```python
from build123d import *

# Parameters (mm, degrees)
REVOLUTION_ANGLE = -357
SKETCH002_R      = 19.5
POCKET_DEPTH     = 36.501
POCKET001_DEPTH  = 15
CHAMFER_SIZE     = 0.25
CHAMFER001_SIZE  = 0.5
CHAMFER002_SIZE  = 0.5
CHAMFER003_SIZE  = 1


with BuildPart() as part:
    # Sketch → Revolution (revolve)
    with BuildSketch(Plane(origin=(0, 0, 0), x_dir=(0, 0, -1), z_dir=(0, -1, 0))):
        Polygon((-36.5, 0), (0, 0), (0, -21.5), (-19.5, -21.5), (-19.5, -26), (-36.5, -26), align=None)
    revolve(axis=Axis((0, 0, 0), (0, 0, -1)), revolution_arc=REVOLUTION_ANGLE)

    # Sketch002 → Pocket (cut, through all)
    with BuildSketch(Plane.XY):
        Circle(SKETCH002_R)
    extrude(amount=POCKET_DEPTH, mode=Mode.SUBTRACT)

    # Sketch001 → Pocket001 (cut)
    with BuildSketch(Plane.XY.offset(36.5)):
        with BuildLine():
            ThreePointArc((-15.975, 16.475), (-16.828553, 16.828553), (-16.475, 15.975))
            Line((-16.475, -15.975), (-16.475, 15.975))
            ThreePointArc((-16.475, -15.975), (-16.828553, -16.828553), (-15.975, -16.475))
            Line((15.975, -16.475), (-15.975, -16.475))
            ThreePointArc((15.975, -16.475), (16.828553, -16.828553), (16.475, -15.975))
            Line((16.475, 15.975), (16.475, -15.975))
            ThreePointArc((16.475, 15.975), (16.828553, 16.828553), (15.975, 16.475))
            Line((15.975, 16.475), (-15.975, 16.475))
        make_face()
    extrude(amount=-POCKET001_DEPTH, mode=Mode.SUBTRACT)

    # Chamfer
    chamfer_edges = [part.edges().sort_by_distance(p)[0] for p in [
        (-16.475, -10.431892, 29),
        (-10.431892, -16.475, 29),
        (10.431892, -16.475, 29),
        (16.475, -10.431892, 29),
        (-16.475, 10.431892, 29),
        (-10.431892, 16.475, 29),
        (10.431892, 16.475, 29),
        (16.475, 10.431892, 29),
    ]]
    chamfer(chamfer_edges, length=CHAMFER_SIZE)

    # Chamfer001
    chamfer001_edges = [part.edges().sort_by_distance(p)[0] for p in [
        (25.99109, -0.680601, 36.5),
    ]]
    chamfer(chamfer001_edges, length=CHAMFER001_SIZE)

    # Chamfer002
    chamfer002_edges = [part.edges().sort_by_distance(p)[0] for p in [
        (25.99109, -0.680601, 19.5),
    ]]
    chamfer(chamfer002_edges, length=CHAMFER002_SIZE)

    # Chamfer003
    chamfer003_edges = [part.edges().sort_by_distance(p)[0] for p in [
        (21.492632, -0.562804, 0),
    ]]
    chamfer(chamfer003_edges, length=CHAMFER003_SIZE)


solid = part.part
```
Source: CAD feature listing. Evaluate the final solid. Frame: model axes, mm. A direction names the side the tool comes from. Coordinates: 2 decimals unless noted, no trailing zeros. Write each loop counter-clockwise with the first axis right and the second up, starting at its lowest first coordinate (ties: lowest second). Pieces come first, ordered by that corner, then holes. Notation, with made-up numbers: (-15, 27.25) -> (9, 27.25) arc R11 cw to (9, 33.25) -> close; hole circle Ø6 at (24, -8.75). An arc over 180 degrees is marked (long way). Return JSON: item names as keys, results as strings. Group by question number.
1) Ray query, line 1 along Y through (x, z) = (0, 12); line 2 along Z through (x, y) = (-22.5, 4.5); line 3 along Y through (x, z) = (15, 31.5) (3 decimals). Return the intervals inside material, ascending.
2) Section query A-A, the plane x = 0. Return loops of the section in (y, z).
3) Mould query, pull axis X, two halves, no side actions, for faces 6 (the face through (13, 16.475, 29)), 7 (the face through (-11, 19, 19.5)), 8 (the face through (-21.95, 1.15, 22.05)). Classes: +X half, -X half, draft (parallel to the pull), parting line (faces both ways), or undercut.
4) Section query B-B, the plane z = 4. Return loops of the section in (x, y).
5) Set-up query: faces 1 (the face through (21.448, -1.499, 10.38)), 2 (the face through (-22, 0, 22)), 3 (the face through (-13, 16.475, 29)), 4 (the face through (17, -10, 36.5)), 5 (the face through (25.937, -1.813, 28.112)). Return all of +Z, -Z, +X, -X, +Y, -Y with unobstructed straight access to the full face (end or side cutting, diameter ignored); none if empty.
6) Contact query for flat-ended pins moving along their axis: P1, Ø2.5, axis at y = -12.5, z = 28.5, coming from the -X side; P2, Ø6, axis at x = -14, z = 30.5, coming from the +Y side; P3, Ø7.5, axis at x = 12, y = 12, coming from the +Z side. Output: stop coordinate, or through.
From the geometry:
{
 "1": {"line 1": "-21.5 to -19.5, 19.5 to 21.5", "line 2": "19.5 to 36.5", "line 3": "-21.237 to -16.475, 16.475 to 21.237"},
 "2": {"outline": "(-26, 20) -> (-25.5, 19.5) -> (-21.5, 19.5) -> (-21.5, 1) -> (-20.5, 0) -> (-19.5, 0) -> (-19.5, 36.5) -> (-25.5, 36.5) -> (-26, 36) -> close; (19.5, 0) -> (20.5, 0) -> (21.5, 1) -> (21.5, 19.5) -> (25.5, 19.5) -> (26, 20) -> (26, 36) -> (25.5, 36.5) -> (19.5, 36.5) -> close"},
 "3": {"face 6": "undercut", "face 7": "draft", "face 8": "-X half"},
 "4": {"outline": "(-21.5, 0) arc R21.5 ccw (long way) to (-21.47, 1.13) -> (-19.47, 1.02) arc R19.5 cw (long way) to (-19.5, 0) -> close"},
 "5": {"face 1": "-Z", "face 2": "+Z, -Z, -X", "face 3": "+Z", "face 4": "+Z, +X, -X, +Y, -Y", "face 5": "+Z, -Z"},
 "6": {"P1": "x = -23.44", "P2": "y = 23.56", "P3": "z = 21.5"}
}
